Verification items for the finished model (mm, model axes). A direction names the side the tool comes from. Round coordinates to 2 decimals unless told otherwise and drop trailing zeros. Loops run counter-clockwise (first coordinate to the right, second up) from the corner with the lowest first, then second, coordinate; pieces in that order, holes last.
from build123d import *

# Parameters (mm, degrees)
REVOLVE1_ANGLE                 = 16
SKETCH4_W                      = 10
SKETCH4_H                      = 5
MAKERBEAMSUPPORT_DEPTH         = 10
SKETCH5_R                      = 1.6
MAKERBEAMHOLE_DEPTH            = 18
MAKERBEAMHOLELINEARRIGHT_COUNT = 2
MAKERBEAMHOLELINEARRIGHT_PITCH = 10
MIRROR3_COPY_1_SKETCH_W        = 10
MIRROR3_COPY_1_SKETCH_H        = 5
MIRROR3_COPY_1_DEPTH           = 10
MIRROR3_COPY_2_SKETCH_R        = 1.6
MIRROR3_COPY_2_DEPTH           = 18
MIRROR3_COPY_3_SKETCH_W        = 10
MIRROR3_COPY_3_SKETCH_H        = 5
MIRROR3_COPY_3_DEPTH           = 10
FILLET7_R                      = 2
SKETCH8_R                      = 1.6
CUT_EXTRUDE8_DEPTH             = 6


with BuildPart() as part:
    # Sketch1 → Revolve1 (revolve, symmetric)
    with BuildSketch(Plane.XY) as revolve1_sk:
        Polygon((98, 17), (98, 0), (116, 0), (116, 5), (108, 5), (108, 17), align=None)
    revolve(axis=Axis((0, -55, 0), (0, 1, 0)), revolution_arc=REVOLVE1_ANGLE / 2)
    revolve(revolve1_sk.sketch, axis=Axis((0, -55, 0), (0, -1, 0)), revolution_arc=REVOLVE1_ANGLE / 2)

    # Sketch4 → MakerBeamSupport (add)
    with BuildSketch(Plane(origin=(111, 0, 0), x_dir=(0, 0, -1), z_dir=(1, 0, 0))):
        with Locations((0, 2.5)):
            Rectangle(SKETCH4_W, SKETCH4_H)
    makerbeamsupport = extrude(amount=MAKERBEAMSUPPORT_DEPTH)

    # Sketch5 → MakerBeamHole (cut, through all)
    with BuildSketch(Plane(origin=(0, 0, 0), x_dir=(-1, 0, 0), z_dir=(0, -1, 0))):
        with Locations((-116, 0)):
            Circle(SKETCH5_R)
    makerbeamhole = extrude(amount=-MAKERBEAMHOLE_DEPTH, mode=Mode.SUBTRACT)

    # MakerBeamHoleLinearRight: MakerBeamSupport, MakerBeamHole ×2
    with Locations(*[(0, 0, -i * MAKERBEAMHOLELINEARRIGHT_PITCH) for i in range(1, MAKERBEAMHOLELINEARRIGHT_COUNT)]):
        add(makerbeamsupport)
        add(makerbeamhole, mode=Mode.SUBTRACT)

    # Mirror3: MakerBeamHole across plane
    add(makerbeamhole.mirror(Plane.XY), mode=Mode.SUBTRACT)

    # Mirror3 copy 1 sketch → Mirror3 copy 1 (add)
    with BuildSketch(Plane(origin=(111, 0, 10), x_dir=(0, 0, 1), z_dir=(1, 0, 0))):
        with Locations((0, -2.5)):
            Rectangle(MIRROR3_COPY_1_SKETCH_W, MIRROR3_COPY_1_SKETCH_H)
    extrude(amount=MIRROR3_COPY_1_DEPTH)

    # Mirror3 copy 2 sketch → Mirror3 copy 2 (cut, through all)
    with BuildSketch(Plane(origin=(0, 0, 10), x_dir=(-1, 0, 0), z_dir=(0, -1, 0))):
        with Locations((-116, 0)):
            Circle(MIRROR3_COPY_2_SKETCH_R)
    extrude(amount=-MIRROR3_COPY_2_DEPTH, mode=Mode.SUBTRACT)

    # Mirror3 copy 3 sketch → Mirror3 copy 3 (add)
    with BuildSketch(Plane(origin=(111, 0, 0), x_dir=(0, 0, 1), z_dir=(1, 0, 0))):
        with Locations((0, -2.5)):
            Rectangle(MIRROR3_COPY_3_SKETCH_W, MIRROR3_COPY_3_SKETCH_H)
    extrude(amount=MIRROR3_COPY_3_DEPTH)

    # Fillet7
    fillet7_edges = [part.edges().sort_by_distance(p)[0] for p in [
        (108, 5, 0),
    ]]
    fillet(fillet7_edges, radius=FILLET7_R)

    # Sketch8 → Cut-Extrude8 (cut, through all)
    with BuildSketch(Plane(origin=(0, 5, 0), x_dir=(1, 0, 0), z_dir=(0, 1, 0))):
        with Locations((116, 0)):
            Circle(SKETCH8_R)
    extrude(amount=-CUT_EXTRUDE8_DEPTH, mode=Mode.SUBTRACT)


solid = part.part
1. Section check C-C (y = 12). Enter the section's corners in (x, z), then the cut area to 3 significant figures.
2. Section check D-D (x = 104). Enter the section's corners in (y, z).
3. Section check B-B (z = 0). Enter the section's corners in (x, y), then the cut area to 3 significant figures.
4. Section check A-A (x = 116). Enter the section's corners in (y, z).
5. Tool access check on faces 4 (the face through (118, 3, 15)), 5 (the face through (103.853, 6.73, 14.596)), 6 (the face through (108, 12, 0)). Record the directions out of +Z, -Z, +X, -X, +Y, -Y that give a thin tool (end or side, any length) a straight path to the whole face; none if there is none.
6. Scan lines: L1, parallel to Z at x = 116, y = 2.8; L2, parallel to X at y = 1.65, z = 0; L3, parallel to Y at x = 109.75, z = 14.5. Record each from-to range of solid material in increasing order.
7. Gauge pin test, flat ends, axial feed: P1, Ø3.5, axis at x = 112, z = 8, coming from the +Y side; P2, Ø6, axis at y = 15, z = 10, coming from the +X side; P3, Ø6, axis at x = 109, y = 7.5, coming from the +Z side. Record the tip position at first contact, or that the pin passes through.
8. Release check for a two-part mould opening along Z. For faces 1 (the face through (121, 2, 0)), 2 (the face through (118, 2, -15)), 3 (the face through (114.474, 2.465, 9.519)) record: released by +Z, released by -Z, zero draft, split by the parting line, or undercut.
Taken from the geometry:
1. outline: (97.05, -13.64) - (106.95, -15.03) arc R108 ccw to (106.95, 15.03) - (97.05, 13.64) arc R98 cw to start
1. area: 288 mm2
2. outline: (0, -14.62) - (17, -14.62) - (17, 14.62) - (0, 14.62) - close
3. outline: (98, 0) - (114.4, 0) - (114.4, 5) - (110, 5) arc R2 cw to (108, 7) - (108, 17) - (98, 17) - close; (117.6, 0) - (121, 0) - (121, 5) - (117.6, 5) - close
3. area: 220 mm2
4. outline: (0, -15) - (5, -15) - (5, -11.6) - (0, -11.6) - close; (0, -8.4) - (5, -8.4) - (5, -1.6) - (0, -1.6) - close; (0, 1.6) - (5, 1.6) - (5, 8.4) - (0, 8.4) - close; (0, 11.6) - (5, 11.6) - (5, 15) - (0, 15) - close
5. face 4: +Z, +X, +Y, -Y
5. face 5: +Z, -X, +Y, -Y
5. face 6: +X, +Y
6. L1: z = -15 to -11.6, -8.4 to -1.6, 1.6 to 8.4, 11.6 to 15
6. L2: x = 98 to 114.4, 117.6 to 121
6. L3: y = 0 to 5
7. P1: stops at y = 5
7. P2: stops at x = 107.77
7. P3: stops at z = 15.55
8. face 1: zero draft
8. face 2: released by -Z
8. face 3: undercut
